The model under review builds one solid part; all positions refer to its coordinate system, in mm. Give positions to 0.01 mm unless a question says otherwise; leave off trailing zeros. Order: outer loops, then holes, each group sorted by start corner. A loop starts at its lowest first (then second) coordinate and runs counter-clockwise, first axis right, second up. Notation, with made-up numbers: M 17,47.5 L 53,47.5 A24 ccw 53,82.5 Z; hole C 37.5,-1 d8. An arc over 180 degrees is marked long. One line per question, with ' | ' between items. Start each with the question number.
1. Wall thickness on L1, parallel to Z at x = 25, y = 1.5; L2, parallel to X at y = 1.6, z = 5; L3, parallel to Z at x = 47, y = 1.45: over which ranges is each line inside the solid? List them lowest first.
2. The part is to be moulded in two halves that separate along Z. For faces 1 (the face through (8.026, 1.014, 39.894)), 2 (the face through (8, 2, 24)), 3 (the face through (48.464, 0.986, 11.675)), 4 (the face through (3.55, 0.99, 5.43)), say which applies: +Z half, -Z half, draft (parallel to the pull), parting line (faces both ways), or undercut.
3. We need section A-A on x = 4. Write out the cut boundary in (y, z), then the cut area to 3 significant figures.
4. We need section B-B on y = 0.5. Write out the cut boundary in (x, z).
5. We need section C-C on z = 4. Write out the cut boundary in (x, y), then the cut area to 3 significant figures.
6. We need section D-D on x = 25. Write out the cut boundary in (y, z).
Autodesk Inventor part; units mm, degrees
ref_plane "YZ Plane" through (0, 0, 0) normal (1, 0, 0) x (0, 1, 0)
ref_plane "XZ Plane" through (0, 0, 0) normal (0, 1, 0) x (-1, 0, 0)
ref_plane "XY Plane" through (0, 0, 0) normal (0, 0, 1) x (1, 0, 0)
sketch "スケッチ8" plane through (0, 0, 0) normal (0, 1, 0) x (-1, 0, 0)
  line L0 (0, 0) -> (-8, -6)
  line L1 (-8, -6) -> (-28, -6)
  line L2 (-28, -6) -> (-50, 11)
  line L3 (-50, 11) -> (-50, 23)
  line L4 (-50, 23) -> (-28, 40)
  line L5 (-28, 40) -> (-8, 40)
  line L6 (-8, 40) -> (0, 34)
  line L7 (0, 34) -> (0, 0)
  circle A0 centre (-25, 17) radius 17.35
  dimension "d41" = 34
  dimension "d42" = 6
  dimension "d43" = 6
  dimension "d44" = 8
  dimension "d45" = 20
  dimension "d46" = 22
  dimension "d47" = 17
  dimension "d48" = 17
  dimension "d49" = 34.7
  dimension "d50" = 25
  dimension "d51" = 23
extrude "プレート6" add sketch "スケッチ8" along normal blind 2
sketch "スケッチ9" plane through (0, 2, 0) normal (0, 1, 0) x (1, 0, 0)
  line L0 (0, -34) -> (0, 0)
  line L1 (50, -11) -> (50, -23)
  point P0 (4, -4)
  point P1 (4, -30)
  point P2 (47, -22)
  point P3 (47, -12)
  dimension "d53" = 4
  dimension "d54" = 4
  dimension "d55" = 26
  dimension "d56" = 3
  dimension "d57" = 1
  dimension "d58" = 1
hole "穴1" at (4, 2, 4) at (4, 2, 30) at (47, 2, 22) at (47, 2, 12) direction (0, -1, 0) diameter 3 end through all
fillet "コーナーR1" radius 2 8 edges at (0, 1, 34) (8, 1, 40) (28, 1, 40) (50, 1, 23) (50, 1, 11) (28, 1, -6) (0, 1, 0) (8, 1, -6)
sketch "スケッチ10" plane through (49.2229, 0, 23.6005) normal (0.6114475, 0, 0.791285) x (0.791285, 0, -0.6114475)
  point P0 (-24.5189, 0)
equation "\"d64\" = Thickness"
equation "\"d52\" = Thickness"
equation "\"BendRadius\" = Thickness"
equation "\"BendReliefWidth\" = Thickness"
equation "\"BendReliefDepth\" = 0.5 * Thickness"
equation "\"CornerReliefSize\" = 4 * Thickness"
equation "\"MinimumRemnant\" = 2 * Thickness"
equation "\"TransitionRadius\" = BendRadius"
equation "\"JacobiRadiusSize\" = Thickness"
equation "\"GapSize\" = Thickness"
properties part number "trackball-cover" material "アルミニウム 6061"
Entries:
1) L1: z = -6 to -0.35, 34.35 to 40 | L2: x = 0 to 2.88, 5.12 to 12.47, 37.53 to 42.24 | L3: z = 8.68 to 10.5, 13.5 to 20.5, 23.5 to 25.32
2) face 1: +Z half | face 2: draft | face 3: undercut | face 4: undercut
3) outline: M 0,-3 L 2,-3 L 2,2.5 L 0,2.5 Z; M 0,5.5 L 2,5.5 L 2,28.5 L 0,28.5 Z; M 0,31.5 L 2,31.5 L 2,37 L 0,37 Z | area: 68.0 mm^2
4) outline: M 0,1 A2 ccw 0.8,-0.6 L 7.47,-5.6 A2 ccw 8.67,-6 L 27.32,-6 A2 ccw 28.54,-5.58 L 49.22,10.4 A2 ccw 50,11.98 L 50,22.02 A2 ccw 49.22,23.6 L 28.54,39.58 A2 ccw 27.32,40 L 8.67,40 A2 ccw 7.47,39.6 L 0.8,34.6 A2 ccw 0,33 Z; hole C 4,4 d3; hole C 4,30 d3; hole C 25,17 d34.7; hole C 47,12 d3; hole C 47,22 d3
5) outline: M 0,0 L 2.5,0 L 2.5,2 L 0,2 Z; M 5.5,0 L 13.51,0 L 13.51,2 L 5.5,2 Z; M 36.49,0 L 40.94,0 L 40.94,2 L 36.49,2 Z | area: 29.9 mm^2
6) outline: M 0,-6 L 2,-6 L 2,-0.35 L 0,-0.35 Z; M 0,34.35 L 2,34.35 L 2,40 L 0,40 Z
